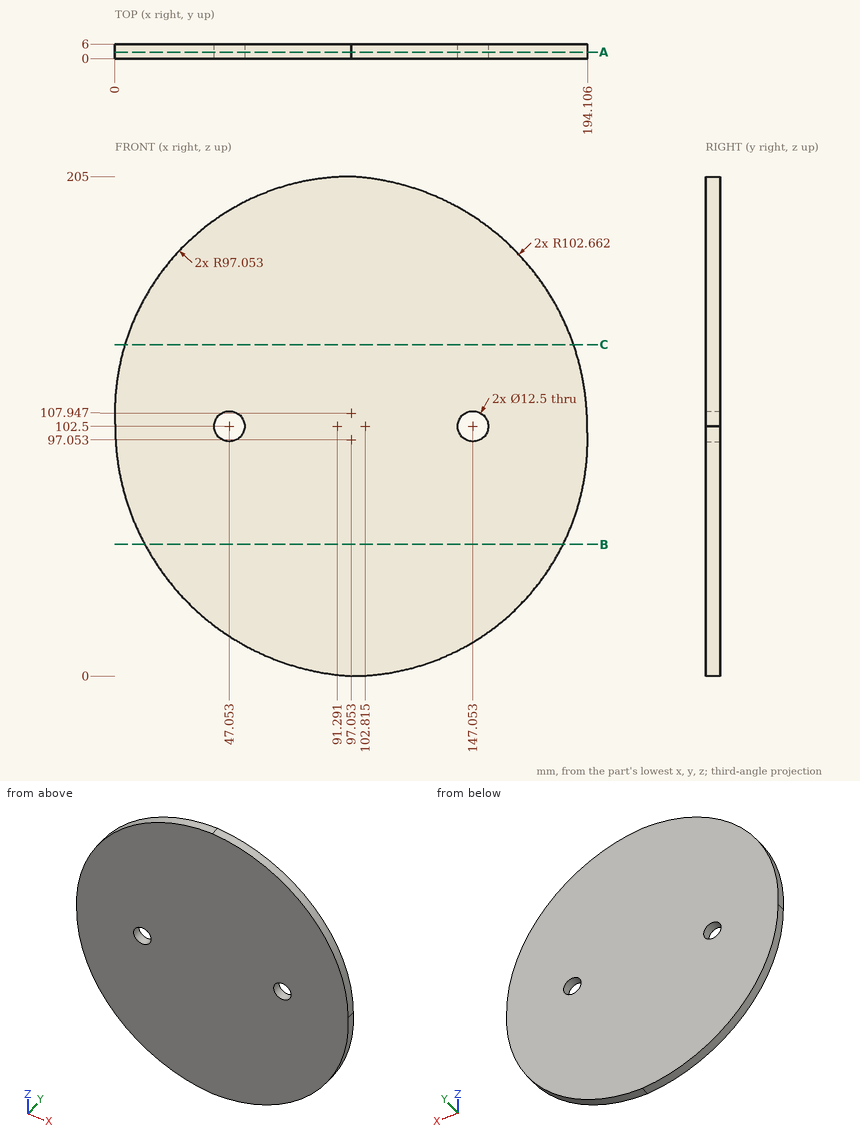
For this review, use the dimensioned drawing (mm, ordinates from the lowest corner) and the shaded views. Coordinates: 2 decimals unless noted, no trailing zeros. Loops run counter-clockwise (first coordinate to the right, second up) from the corner with the lowest first, then second, coordinate; pieces in that order, holes last. Notation, with made-up numbers: (-30, 63.5) -> (21, 63.5) arc R16 ccw to (21, 93.5) -> close; hole circle Ø3 at (45.25, 80). An arc over 180 degrees is marked (long way). Use a Markdown table: item, result. Add a question column.
Item 1: Clearance check with flat-ended pins moving along their axes: P1, Ø1, axis at x = 106, z = 97.5, coming from the -Y side; P2, Ø2, axis at y = 3, z = 126, coming from the +X side; P3, Ø1.5, axis at y = 3, z = 164.5, coming from the +X side. State where each tip first meets the part, or that it passes through.
Item 2: Wall thickness on L1, parallel to X at y = 2.8, z = 102.5; L2, parallel to Z at x = 14, y = 1.9; L3, parallel to Z at x = 85, y = 2.7: over which ranges is each line inside the solid? List them lowest first. Write a range as from..to.
Item 3: We need section A-A, the plane y = 2.65. Count the separate pieces of the cut face and the enclosed holes in it, and give its area (3 significant figures).
Item 4: We need section C-C, the plane z = 136. Write out the cut boundary in (x, y), and give its area (4 significant figures).
Item 5: We need section B-B, the plane z = 54. Write out the cut boundary in (x, y), and give its area (3 significant figures).
Numbers:
| question | item | result |
|---|---|---|
| 1 | P1 | stops at y = 0 |
| 1 | P2 | stops at x = 191.46 |
| 1 | P3 | stops at x = 173.68 |
| 2 | L1 | x = 0.15..40.8, 53.3..140.8, 153.3..193.95 |
| 2 | L2 | z = 51.01..158.16 |
| 2 | L3 | z = 1.4..204.25 |
| 3 | separate pieces | 1 |
| 3 | enclosed holes | 2 |
| 3 | area | 31,000 mm^2 |
| 4 | outline | (4.14, 0) -> (188.33, 0) -> (188.33, 6) -> (4.14, 6) -> close |
| 4 | area | 1,105 mm^2 |
| 5 | outline | (12.33, 0) -> (184.03, 0) -> (184.03, 6) -> (12.33, 6) -> close |
| 5 | area | 1,030 mm^2 |
